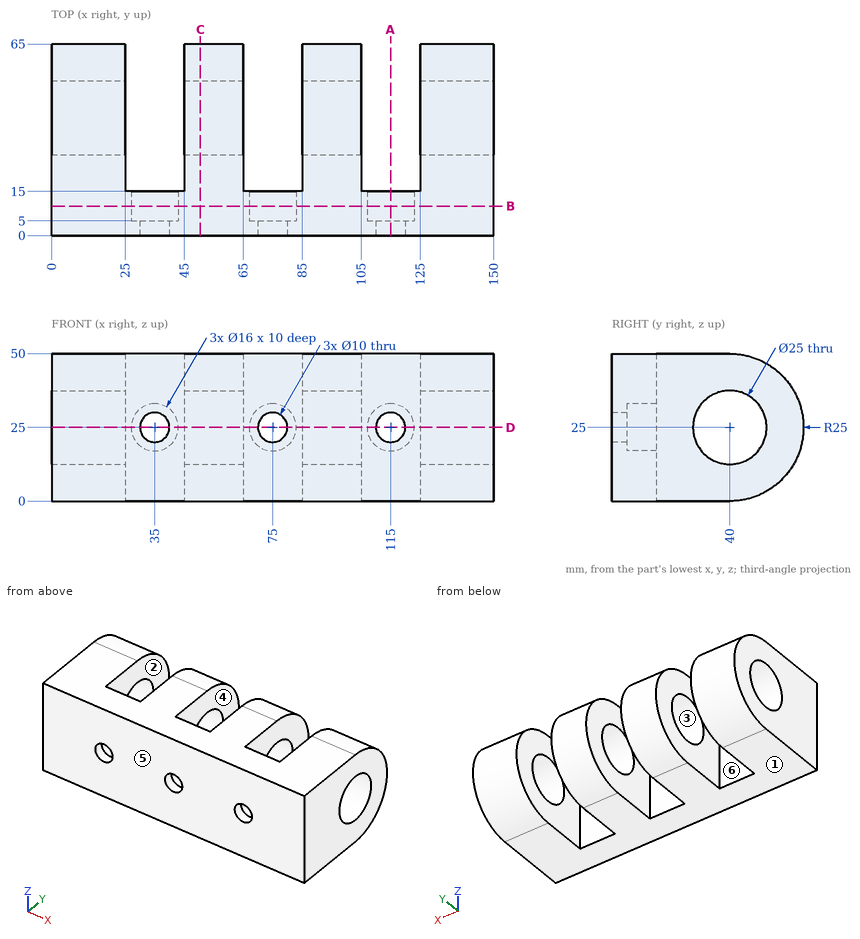
Input: dimensioned drawing with shaded views. Units: mm. Origin: part minimum x, y, z. A direction names the side the tool comes from. Round coordinates to 2 decimals unless told otherwise and drop trailing zeros. Loops run counter-clockwise (first coordinate to the right, second up) from the corner with the lowest first, then second, coordinate; pieces in that order, holes last. Notation, with made-up numbers: (68, -38) -> (93, -38) arc R23 cw to (93, -26) -> close; hole circle Ø6 at (59, 88.25). An arc over 180 degrees is marked (long way). Answer as a JSON object with one key per item and string values. Group by question number.
Q1. Ray query, line 1 (X direction, y = 10, z = 25); line 2 (X direction, y = 3.4, z = 25); line 3 (Y direction, x = 58.25, z = 25). Return the intervals inside material, ascending. Write a range as from..to.
Q2. Mould query, pull axis Y, two halves, no side actions, for the marked faces 3, 4, 5 and 6. Classes: pulls with the +Y half, pulls with the -Y half, needs draft (parallel to the pull), parting line crosses it, or undercut.
Q3. Section query B-B (y = 10). Output: boundary loops of the cut face in (x, z).
Q4. Access query for the marked faces 1 and 2. Directions: +Z, -Z, +X, -X, +Y, -Y. A direction counts if a zero-diameter tool reaches every point of the face in a straight line with its end or side. Return the directions, or none.
Q5. Contact query for flat-ended pins moving along their axis: P1, Ø11.5, axis at x = 75, z = 25, coming from the +Y side; P2, Ø2, axis at x = 55, y = 44, coming from the +Z side; P3, Ø13, axis at x = 74, z = 26.5, coming from the +Y side; P4, Ø6, axis at x = 35, z = 25, coming from the -Y side. Output: stop coordinate, or through.
Q6. Section query D-D (z = 25). State how many separate pieces and enclosed holes the cut face has, plus the area to 3 significant figures.
Q7. Section query A-A (x = 115). Output: boundary loops of the cut face in (y, z).
Q8. Section query C-C (x = 50.5). Output: boundary loops of the cut face in (y, z).
Completed:
{
 "1": {"line 1": "0..27, 43..67, 83..107, 123..150", "line 2": "0..30, 40..70, 80..110, 120..150", "line 3": "0..27.5, 52.5..65"},
 "2": {"face 3": "undercut", "face 4": "needs draft", "face 5": "pulls with the -Y half", "face 6": "pulls with the +Y half"},
 "3": {"outline": "(0, 0) -> (150, 0) -> (150, 50) -> (0, 50) -> close; hole circle Ø16 at (35, 25); hole circle Ø16 at (75, 25); hole circle Ø16 at (115, 25)"},
 "4": {"face 1": "-Z, +X, -X, +Y, -Y", "face 2": "+Z, -Z, +Y"},
 "5": {"P1": "y = 5", "P2": "z = 49.82", "P3": "y = 15", "P4": "through"},
 "6": {"separate pieces": "8", "enclosed holes": "0", "area": "3,870 mm²"},
 "7": {"outline": "(0, 0) -> (15, 0) -> (15, 17) -> (5, 17) -> (5, 20) -> (0, 20) -> close; (0, 30) -> (5, 30) -> (5, 33) -> (15, 33) -> (15, 50) -> (0, 50) -> close"},
 "8": {"outline": "(0, 0) -> (40, 0) arc R25 ccw to (40, 50) -> (0, 50) -> close; hole circle Ø25 at (40, 25)"}
}
